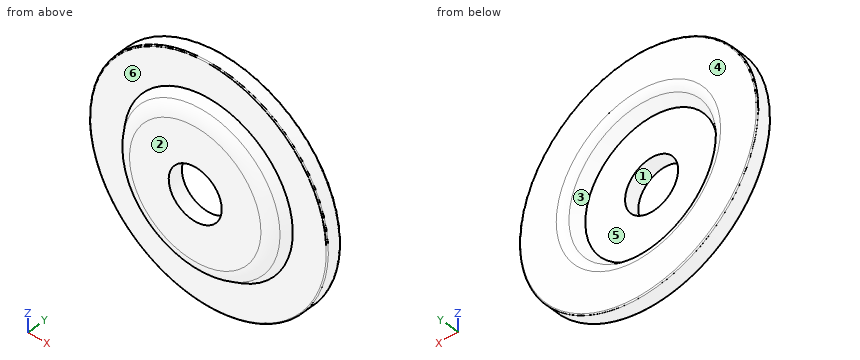
```python
from build123d import *


with BuildPart() as part:
    # Sketch1 → Revolve1 (revolve)
    with BuildSketch(Plane.XY, mode=Mode.PRIVATE) as revolve1_sk:
        with BuildLine():
            Line((2.5, 0), (6.25, 0))
            Line((6.25, 0), (6.930508845, 0.973091831))
            ThreePointArc((6.930508845, 0.973091831), (7.287989086, 1.286874239), (7.75, 1.4))
            Line((7.75, 1.4), (11.125, 1.4))
            ThreePointArc((11.125, 1.4), (11.195710678, 1.370710678), (11.225, 1.3))
            Line((11.225, 1.3), (11.225, 0.1))
            ThreePointArc((11.225, 0.1), (11.195710678, 0.029289322), (11.125, 0))
            Line((11.125, 0), (7.958377194, 0))
            Line((7.958377194, 0), (7.427142434, -0.759637747))
            ThreePointArc((7.427142434, -0.759637747), (6.890922072, -1.230311358), (6.197905701, -1.4))
            Line((6.197905701, -1.4), (2.5, -1.4))
            Line((2.5, -1.4), (2.5, 0))
        make_face()
    revolve(revolve1_sk.sketch.rotate(Axis((0, 11.539064392, 0), (0, -1, 0)), 90), axis=Axis((0, 11.539064392, 0), (0, -1, 0)))


solid = part.part
```
Verification items for the finished model (mm, model axes). Face numbers are marked on the shaded views. A direction names the side the tool comes from. Coordinates: 2 decimals unless noted, no trailing zeros. Write each loop counter-clockwise with the first axis right and the second up, starting at its lowest first coordinate (ties: lowest second). Pieces come first, ordered by that corner, then holes. Notation, with made-up numbers: M 11.5,-19.75 L 63.5,-19.75 A12 ccw 63.5,-12.75 Z; hole C -17,0 d5. An arc over 180 degrees is marked long. One line per item, written item: value.
Item 1: Access from +Z, -Z, +X, -X, +Y, -Y to the whole of each face (thin tool, end or side, straight path). Record for the marked faces 4, 5 and 6.
Check sheet entries:
face 4: +Z, -Z, +X, -X, +Y
face 5: +Y
face 6: -Y
Item 2: Gauge pin test, flat ends, axial feed: pin 1 Ø1.5 at (x, z) = (6.5, 1) entering from +Y; pin 2 Ø4 at (x, z) = (-4.5, 4) entering from +Y; pin 3 Ø1 at (y, z) = (0, 5.5) entering from +X; pin 4 Ø1 at (y, z) = (0, 7) entering from -X. Record the tip position at first contact, or that the pin passes through.
Check sheet entries:
pin 1: stops at y = 1.31
pin 2: stops at y = 1.4
pin 3: stops at x = 10.05
pin 4: stops at x = -9.15
Item 3: Section check C-C, the plane y = 0.55. Record the boundary of the cut face in (x, z) (3 decimals).
Check sheet entries:
outline: C 0,0 d22.45; hole C 0,0 d13.269
Item 4: Scan lines: line 1 along Y through (x, z) = (-5.5, 0.75); line 2 along Z through (x, y) = (-2, -0.1); line 3 along X through (y, z) = (-0.9, 0). Record each from-to range of solid material in increasing order.
Check sheet entries:
line 1: y = -1.4 to 0
line 2: z = -7.63 to -1.5, 1.5 to 7.63
line 3: x = -7.32 to -2.5, 2.5 to 7.32
Item 5: Mould release check, pull along Z, two halves, no side actions. Record for the marked faces 1, 2 and 3: pulls with the +Z half, pulls with the -Z half, needs draft (parallel to the pull), parting line crosses it, or undercut.
Check sheet entries:
face 1: undercut
face 2: needs draft
face 3: undercut
